Could you check a few things on this model? Use its own coordinates, in mm. Give positions to 0.01 mm unless a question says otherwise; leave off trailing zeros. Order: outer loops, then holes, each group sorted by start corner. A loop starts at its lowest first (then second) coordinate and runs counter-clockwise, first axis right, second up. Notation, with made-up numbers: (28, -35.5) -> (70, -35.5) arc R12 cw to (70, -17.5) -> close; hole circle Ø5 at (18, 63). An arc over 180 degrees is marked (long way). Write each question's results on one line, items separated by ' | '.
```python
from build123d import *

# Parameters (mm, degrees)
SKETCH1_W               = 164.9
SKETCH1_H               = 114.9
BOSS_EXTRUDE1_DEPTH     = 1.5
SKETCH2_R               = 1.75
BOSS_EXTRUDE2_DEPTH     = 1.5
LPATTERN1_COUNT         = 2
LPATTERN1_PITCH         = 100.8
MIRROR1_COPY_1_SKETCH_R = 1.75
MIRROR1_COPY_1_DEPTH    = 1.5


with BuildPart() as part:
    # Sketch1 → Boss-Extrude1 (new body)
    with BuildSketch(Plane(origin=(0, 0, 0), x_dir=(1, 0, 0), z_dir=(0, 1, 0))):
        Rectangle(SKETCH1_W, SKETCH1_H)
    extrude(amount=BOSS_EXTRUDE1_DEPTH)

    # Sketch2 → Boss-Extrude2 (add)
    with BuildSketch(Plane(origin=(0, 1.5, 0), x_dir=(1, 0, 0), z_dir=(0, 1, 0))):
        with BuildLine():
            Line((-82.45, 55.65), (-82.45, 45.15))
            Line((-82.45, 45.15), (-86.45, 45.15))
            ThreePointArc((-86.45, 45.15), (-91.7, 50.4), (-86.45, 55.65))
            Line((-86.45, 55.65), (-82.45, 55.65))
        make_face()
        with Locations(Location((-86.45, 50.4, 0), (0, 0, 270))):
            Circle(SKETCH2_R, mode=Mode.SUBTRACT)
    boss_extrude2 = extrude(amount=-BOSS_EXTRUDE2_DEPTH)

    # LPattern1: Boss-Extrude2 ×2
    with Locations(*[(0, 0, i * LPATTERN1_PITCH) for i in range(1, LPATTERN1_COUNT)]):
        add(boss_extrude2)

    # Mirror1: Boss-Extrude2 across plane
    add(boss_extrude2.mirror(Plane(origin=(0, 0, 0), x_dir=(0, 0, 1), z_dir=(1, 0, 0))))

    # Mirror1 copy 1 sketch → Mirror1 copy 1 (add)
    with BuildSketch(Plane(origin=(0, 1.5, 100.8), x_dir=(-1, 0, 0), z_dir=(0, 1, 0))):
        with BuildLine():
            Line((-82.45, -55.65), (-82.45, -45.15))
            Line((-82.45, -45.15), (-86.45, -45.15))
            ThreePointArc((-86.45, -45.15), (-91.7, -50.4), (-86.45, -55.65))
            Line((-86.45, -55.65), (-82.45, -55.65))
        make_face()
        with Locations((-86.45, -50.4)):
            Circle(MIRROR1_COPY_1_SKETCH_R, mode=Mode.SUBTRACT)
    extrude(amount=-MIRROR1_COPY_1_DEPTH)


solid = part.part
```
Q1. I'm going to push flat-ended pins straight in: pin 1 Ø0.8 at (y, z) = (1, -57) entering from +X; pin 2 Ø3 at (x, z) = (-86.45, 50.4) entering from +Y; pin 3 Ø0.8 at (y, z) = (1, -56.5) entering from -X; pin 4 Ø0.8 at (x, y) = (84.5, 0.5) entering from -Z. Where does each tip first touch, or does it pass through?
Here are the results:
pin 1: stops at x = 82.45 | pin 2: passes through | pin 3: stops at x = -82.45 | pin 4: stops at z = -55.65
Q2. Suppose I cut it at B-B on y = 0.25. Please give me the cut outline in (x, z).
Here are the results:
outline: (-86.45, -55.65) -> (-82.45, -55.65) -> (-82.45, -57.45) -> (82.45, -57.45) -> (82.45, -55.65) -> (86.45, -55.65) arc R5.25 ccw to (86.45, -45.15) -> (82.45, -45.15) -> (82.45, 45.15) -> (86.45, 45.15) arc R5.25 ccw to (86.45, 55.65) -> (82.45, 55.65) -> (82.45, 57.45) -> (-82.45, 57.45) -> (-82.45, 55.65) -> (-86.45, 55.65) arc R5.25 ccw to (-86.45, 45.15) -> (-82.45, 45.15) -> (-82.45, -45.15) -> (-86.45, -45.15) arc R5.25 ccw to start; hole circle Ø3.5 at (-86.45, -50.4); hole circle Ø3.5 at (-86.45, 50.4); hole circle Ø3.5 at (86.45, -50.4); hole circle Ø3.5 at (86.45, 50.4)
Q3. Thinking about a two-plate mould opening in X: for faces 1 (the flat face through (-1, 0, -1)), 2 (the cylindrical face through (-86.37, 0.76, 48.65)), 3 (the cylindrical face through (91.7, 0.8, 50.5)), which applies, +X half, -X half, draft (parallel to the pull), parting line (faces both ways), or undercut?
Here are the results:
face 1: draft | face 2: undercut | face 3: +X half
Q4. Suppose I cut it at A-A on z = 50.4. Please give me the cut outline in (x, y), and give its area (3 significant figures).
Here are the results:
outline: (-91.7, 0) -> (-88.2, 0) -> (-88.2, 1.5) -> (-91.7, 1.5) -> close; (-84.7, 0) -> (84.7, 0) -> (84.7, 1.5) -> (-84.7, 1.5) -> close; (88.2, 0) -> (91.7, 0) -> (91.7, 1.5) -> (88.2, 1.5) -> close | area: 265 mm²
Q5. I need wall thicknesses on line 1 along Z through (x, y) = (86.45, 0.75); line 2 along X through (y, z) = (1, -50.4); line 3 along X through (y, z) = (1.1, -11). Which ranges of each line are inside material? Lowest first, please.
Here are the results:
line 1: z = -55.65 to -52.15, -48.65 to -45.15, 45.15 to 48.65, 52.15 to 55.65 | line 2: x = -91.7 to -88.2, -84.7 to 84.7, 88.2 to 91.7 | line 3: x = -82.45 to 82.45
Q6. Suppose I cut it at C-C on z = -17. Please give me the cut outline in (x, y).
Here are the results:
outline: (-82.45, 0) -> (82.45, 0) -> (82.45, 1.5) -> (-82.45, 1.5) -> close
